Here's how the part is built. I have some questions about the finished solid (model axes, mm). Face numbers are marked on the shaded views. A direction names the side the tool comes from. Give positions to 0.01 mm unless a question says otherwise; leave off trailing zeros. Order: outer loops, then holes, each group sorted by start corner. A loop starts at its lowest first (then second) coordinate and runs counter-clockwise, first axis right, second up. Notation, with made-up numbers: M 24,-19 L 68,-19 A22 ccw 68,-4 Z; hole C 85.5,84 d2. An arc over 180 degrees is marked long. Use one line per item in the form item = value.
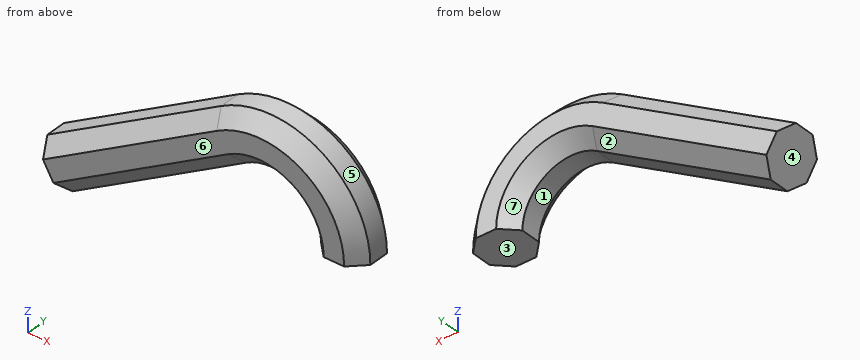
from build123d import *


with BuildPart() as f15:
    # F15: sweep along a path in F14
    with BuildLine(Plane.XZ) as f15_path:
        ThreePointArc((0, 0), (-23.231615305, 39.9364087047), (-69.4313943386, 39.4835211337))
        Line((-69.4313943386, 39.4835211337), (-177.3874624529, -24.7406701782))
    # F13 (on Top) → F15 (sweep)
    with BuildSketch(Plane.XY):
        Polygon((6.35, 15.3302561211), (-6.35, 15.3302561211), (-15.3302561211, 6.35), (-15.3302561211, -6.35), (-6.35, -15.3302561211), (6.35, -15.3302561211), (15.3302561211, -6.35), (15.3302561211, 6.35), align=None)
    sweep(path=f15_path.line)


solid = f15.part
Q1. I want a section at A-A on y = 2. Write out the boundary of the cut face in (x, z).
Found:
outline = M -185.23,-11.57 L -169.55,-37.92 L -61.59,26.31 A30.61 cw -15.33,0 L 15.33,0 A61.27 ccw -77.27,52.66 Z
Q2. I want a section at C-C on z = -22.5. Write out the boundary of the cut face in (x, y).
Found:
outline = M -178.72,-15.33 L -161.2,-15.33 L -143.64,-6.35 L -143.64,6.35 L -161.2,15.33 L -178.72,15.33 Z
Q3. I want a section at B-B on x = -140.5. Write out the boundary of the cut face in (y, z), then the cut area to 3 significant figures.
Found:
outline = M -15.33,-10.18 L -6.35,-20.63 L 6.35,-20.63 L 15.33,-10.18 L 15.33,4.59 L 6.35,15.04 L -6.35,15.04 L -15.33,4.59 Z
area = 906 mm²
Q4. I'm going to push flat-ended pins straight in: pin 1 Ø3 at (x, y) = (-62, -2) entering from +Z; pin 2 Ø10 at (y, z) = (-8, -21) entering from +X; pin 3 Ø8 at (x, y) = (-68, -10.5) entering from -Z. Where does each tip first touch, or does it pass through?
Found:
pin_1 = 59.52
pin_2 = -133.18
pin_3 = 22.1
Q5. Thinking about a two-plate mould opening in X: for the marked faces 4, 5, 6 and 7, which applies, +X half, -X half, draft (parallel to the pull), parting line (faces both ways), or undercut?
Found:
face_4 = -X half
face_5 = parting line
face_6 = draft
face_7 = undercut
Q6. I need wall thicknesses on L1, parallel to X at y = 9.5, z = 15; L2, parallel to X at y = 8, z = 5; L3, parallel to Z at x = -79, y = -12.5. Which ranges of each line are inside material? Lowest first, please.
Found:
L1 = -134.41 to -86.76, -15.7 to 10.21
L2 = -154.15 to -100.64, -14.07 to 13.47
L3 = 23.11 to 44.47
Q7. I want a section at D-D on z = -7. Write out the boundary of the cut face in (x, y).
Found:
outline = M -177.55,-6.35 L -159.99,-15.33 L -135.15,-15.33 L -117.58,-6.35 L -117.58,6.35 L -135.15,15.33 L -159.99,15.33 L -177.55,6.35 Z
Q8. On a 3-axis mill with a long thin cutter (end or side, diameter ignored), from which of +Z, -Z, +X, -X, +Y, -Y can I reach the whole of each face in a straight line? I mean the marked faces 1, 2 and 3. Say none if no direction works.
Found:
face_1 = -Z, +Y, -Y
face_2 = -Z, +Y
face_3 = -Z, +X, +Y, -Y
